For this review, take the finished solid that the model builds, in its own axes (mm). Round coordinates to 2 decimals unless told otherwise and drop trailing zeros. Order: outer loops, then holes, each group sorted by start corner. A loop starts at its lowest first (then second) coordinate and runs counter-clockwise, first axis right, second up. Notation, with made-up numbers: (-2.75, -31.5) - (52.25, -31.5) arc R7 ccw to (52.25, -22.5) - close; hole circle Ø2 at (36, 68). An arc over 180 degrees is marked (long way). One line per item, written item: value.
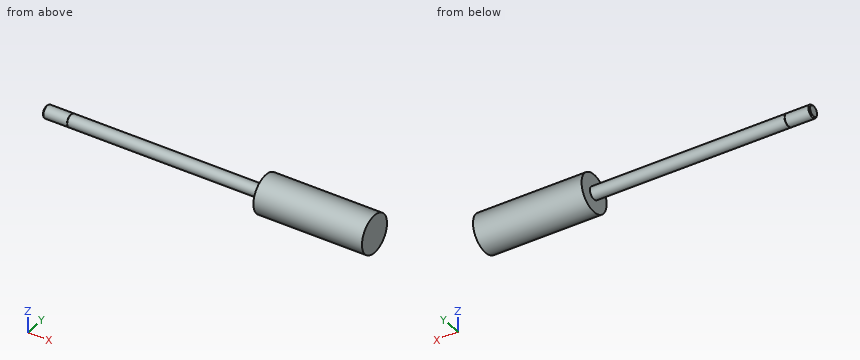
Autodesk Inventor part; units mm, degrees
ref_plane "rod_cp_XY" through (0, 0, 0) normal (1, 0, 0) x (0, 0, -1)
ref_plane "rod_cp_YZ" through (0, 0, 0) normal (0, 0, -1) x (0, 1, 0)
ref_plane "rod_cp_ZX" through (0, 0, 0) normal (0, 1, 0) x (1, 0, 0)
sketch "Sketch_1" plane through (0, 0, 0) normal (0, 0, 1) x (1, 0, 0)
  line L0 (153.3906, 0) -> (0, 0)
  line L1 (0, 0) -> (0, 3.175)
  line L2 (0, 3.175) -> (98.425, 3.175)
  line L3 (98.425, 3.175) -> (98.425, 9.6203)
  line L4 (98.425, 9.6203) -> (153.3906, 9.6203)
  line L5 (153.3906, 9.6203) -> (153.3906, 0)
  line L6 (153.3906, 0) -> (0, 0)
revolve "Revolution1" add sketch "Sketch_1" angle 360 about axis through (153.3906, 0, 0) along (1, 0, 0)
sketch "Sketch_3" plane through (0, 0, 0) normal (0, 0, 1) x (1, 0, 0)
  line L0 (0, 0) -> (-12.7, 0)
  line L1 (-12.7, 0) -> (-12.7, 2.634)
  line L2 (-12.7, 2.634) -> (-12.159, 3.175)
  line L3 (-12.159, 3.175) -> (0, 3.175)
  line L4 (0, 3.175) -> (0, 0)
  line L5 (0, 0) -> (-12.7, 0)
revolve "Revolution2" add sketch "Sketch_3" angle 360 about axis through (0, 0, 0) along (1, 0, 0)
sketch "Sketch_30" plane through (0, 0, 0) normal (0, 0, 1) x (1, 0, 0)
  line L0 (0, 0) -> (-0.254, 0)
  line L1 (-0.254, 3.429) -> (-0.254, 2.921)
  line L2 (-0.254, 2.921) -> (0, 2.921)
  line L3 (0, 2.921) -> (0, 3.429)
  line L4 (0, 3.429) -> (-0.254, 3.429)
revolve "Revolution3" cut sketch "Sketch_30" angle 360 about axis through (0, 0, 0) along (1, 0, 0)
ref_plane "rod_cp_XY" through (0, 0, 0) normal (1, 0, 0) x (0, 0, -1)
ref_plane "rod_cp_YZ" through (0, 0, 0) normal (0, 0, -1) x (0, 1, 0)
ref_plane "rod_cp_ZX" through (0, 0, 0) normal (0, 1, 0) x (1, 0, 0)
ref_plane "to_rod_clevis_XY" through (-12.7, 0, 0) normal (1, 0, 0) x (0, 0, -1)
ref_plane "to_rod_clevis_YZ" through (-12.7, 0, 0) normal (0, 0, -1) x (0, 1, 0)
ref_plane "to_rod_clevis_ZX" through (-12.7, 0, 0) normal (0, 1, 0) x (1, 0, 0)
ref_plane "rl2_XY" through (0, 0, 0) normal (1, 0, 0) x (0, 0, -1)
ref_plane "rl2_YZ" through (0, 0, 0) normal (0, 0, -1) x (0, 1, 0)
ref_plane "rl2_ZX" through (0, 0, 0) normal (0, 1, 0) x (1, 0, 0)
ref_plane "rl1_XY" through (-12.7, 0, 0) normal (1, 0, 0) x (0, 0, -1)
ref_plane "rl1_YZ" through (-12.7, 0, 0) normal (0, 0, -1) x (0, 1, 0)
ref_plane "rl1_ZX" through (-12.7, 0, 0) normal (0, 1, 0) x (1, 0, 0)
ref_plane "thd1_XY" through (-12.7, 3.175, 0) normal (1, 0, 0) x (0, 0, -1)
ref_plane "thd1_YZ" through (-12.7, 3.175, 0) normal (0, 0, -1) x (0, 1, 0)
ref_plane "thd1_ZX" through (-12.7, 3.175, 0) normal (0, 1, 0) x (1, 0, 0)
ref_plane "thd2_XY" through (-12.7, -3.175, 0) normal (1, 0, 0) x (0, 0, -1)
ref_plane "thd2_YZ" through (-12.7, -3.175, 0) normal (0, 0, -1) x (0, 1, 0)
ref_plane "thd2_ZX" through (-12.7, -3.175, 0) normal (0, 1, 0) x (1, 0, 0)
ref_plane "dia1_XY" through (0, 3.175, 0) normal (1, 0, 0) x (0, 0, -1)
ref_plane "dia1_YZ" through (0, 3.175, 0) normal (0, 0, -1) x (0, 1, 0)
ref_plane "dia1_ZX" through (0, 3.175, 0) normal (0, 1, 0) x (1, 0, 0)
ref_plane "dia2_XY" through (0, -3.175, 0) normal (1, 0, 0) x (0, 0, -1)
ref_plane "dia2_YZ" through (0, -3.175, 0) normal (0, 0, -1) x (0, 1, 0)
ref_plane "dia2_ZX" through (0, -3.175, 0) normal (0, 1, 0) x (1, 0, 0)
ref_plane "dia12_XY" through (0, 0, 10.2235) normal (1, 0, 0) x (0, 0, -1)
ref_plane "dia12_YZ" through (0, 0, 10.2235) normal (0, 0, -1) x (0, 1, 0)
ref_plane "dia12_ZX" through (0, 0, 10.2235) normal (0, 1, 0) x (1, 0, 0)
ref_plane "dia22_XY" through (0, 0, -10.2235) normal (1, 0, 0) x (0, 0, -1)
ref_plane "dia22_YZ" through (0, 0, -10.2235) normal (0, 0, -1) x (0, 1, 0)
ref_plane "dia22_ZX" through (0, 0, -10.2235) normal (0, 1, 0) x (1, 0, 0)
properties part number "0430_rod"
Item 1: Take a section at C-C (z = 7). Write out the cut boundary in (x, y) (3 decimals), plus the area to 3 significant figures.
Returned:
outline: (98.425, -6.599) - (153.391, -6.599) - (153.391, 6.599) - (98.425, 6.599) - close
area: 725 mm^2
Item 2: Take a section at B-B (x = 17). Write out the cut boundary in (y, z) (3 decimals).
Returned:
outline: circle Ø6.35 at (0, 0)
Item 3: Wall thickness on line 1 (Y direction, x = 35, z = -1.25); line 2 (X direction, y = 7, z = -3.5) (3 decimals); line 3 (Y direction, x = 30.5, z = 0.25): over which ranges is each line inside the solid? List them lowest first.
Returned:
line 1: -2.92 to 2.92
line 2: 98.425 to 153.391
line 3: -3.17 to 3.17
Item 4: For P1, Ø10, axis at x = 53, z = 4.5, coming from the -Y side (3 decimals); P2, Ø2, axis at x = 70, y = 1, coming from the +Z side (3 decimals); P3, Ø10, axis at x = 79, y = 5.5, coming from the +Z side; P4, Ø10, axis at x = 98, z = 2, coming from the +Y side, all flat-tipped, find the tip position at first contact; note any pin that passes through.
Returned:
P1: y = -3.175
P2: z = 3.175
P3: z = 3.14
P4: y = 9.62
Item 5: Take a section at D-D (y = 7.5). Write out the cut boundary in (x, z) (3 decimals), plus the area to 3 significant figures.
Returned:
outline: (98.425, -6.025) - (153.391, -6.025) - (153.391, 6.025) - (98.425, 6.025) - close
area: 662 mm^2
Item 6: Take a section at A-A (y = 0). Write out the cut boundary in (x, z) (3 decimals).
Returned:
outline: (-12.7, -2.634) - (-12.159, -3.175) - (-0.254, -3.175) - (-0.254, -2.921) - (0, -2.921) - (0, -3.175) - (98.425, -3.175) - (98.425, -9.62) - (153.391, -9.62) - (153.391, 9.62) - (98.425, 9.62) - (98.425, 3.175) - (0, 3.175) - (0, 2.921) - (-0.254, 2.921) - (-0.254, 3.175) - (-12.159, 3.175) - (-12.7, 2.634) - close
